The listing builds one solid part. Answer for the finished solid, in the listing's coordinates (mm). Round coordinates to 2 decimals unless told otherwise and drop trailing zeros. Order: outer loops, then holes, each group sorted by start corner. A loop starts at its lowest first (then second) coordinate and runs counter-clockwise, first axis right, second up. Notation, with made-up numbers: (-37.5, -34.75) -> (16.5, -34.75) arc R19 cw to (16.5, -7.75) -> close; hole circle Ø9 at (63.5, -33). An arc over 180 degrees is marked (long way). Answer in a Markdown table with one row per item. Add a question column.
```python
from build123d import *

# Parameters (mm, degrees)
F0_R     = 1.5875
F0_W     = 152.4
F0_H     = 3.175
F1_DEPTH = 3.175
F2_DEPTH = 6.35
F3_DEPTH = 12.7


# Not quite as in the source:
# - a feature names something its author has since deleted; it is built from what else it names


with BuildPart() as f1:
    # F0 (on Top) → F1 (new body)
    with BuildSketch(Plane.XY):
        with BuildLine():
            Line((76.2, -63.5), (76.2, 60.325))
            Line((76.2, 60.325), (-76.2, 60.325))
            Line((-76.2, 60.325), (-76.2, -63.5))
            Line((-76.2, -63.5), (-76.2, -73.025))
            Line((-76.2, -73.025), (-12.7, -73.025))
            ThreePointArc((-12.7, -73.025), (0, -85.725), (12.7, -73.025))
            Line((12.7, -73.025), (76.2, -73.025))
            Line((76.2, -73.025), (76.2, -63.5))
        make_face()
        with Locations((0, -73.025)):
            Circle(F0_R, mode=Mode.SUBTRACT)
        Polygon((3.175, -50.8), (0, -63.5), (-3.175, -50.8), align=None, mode=Mode.SUBTRACT)
        with BuildLine():
            ThreePointArc((-49.8535963292, 27.0824817792), (-54.4870485305, 34.7644782938), (-46.0375, 31.75))
            ThreePointArc((-46.0375, 31.75), (-46.7742676703, 29.2054203766), (-48.7566120041, 27.4481432208))
            ThreePointArc((-48.7566120041, 27.4481432208), (-45.0579989552, 28.2917059724), (-41.275, 28.575))
            Line((-41.275, 28.575), (41.275, 28.575))
            ThreePointArc((41.275, 28.575), (45.0579989552, 28.2917059724), (48.7566120041, 27.4481432208))
            ThreePointArc((48.7566120041, 27.4481432208), (48.2554203766, 35.7757323297), (55.5625, 31.75))
            ThreePointArc((55.5625, 31.75), (53.8144782938, 28.0629514695), (49.8535963292, 27.0824817792))
            ThreePointArc((49.8535963292, 27.0824817792), (62.0482562055, 17.7911495141), (66.675, 3.175))
            Line((66.675, 3.175), (66.675, -15.875))
            ThreePointArc((66.675, -15.875), (63.3002757063, -28.525977435), (54.0728559007, -37.8152571622))
            ThreePointArc((54.0728559007, -37.8152571622), (55.1742646512, -39.3915948361), (55.5625, -41.275))
            ThreePointArc((55.5625, -41.275), (50.5724196506, -46.0320593264), (46.0592502637, -40.8203592761))
            ThreePointArc((46.0592502637, -40.8203592761), (43.6779018277, -41.1610843708), (41.275, -41.275))
            Line((41.275, -41.275), (-41.275, -41.275))
            ThreePointArc((-41.275, -41.275), (-43.6779018277, -41.1610843708), (-46.0592502637, -40.8203592761))
            ThreePointArc((-46.0592502637, -40.8203592761), (-46.0429406736, -41.0474196506), (-46.0375, -41.275))
            ThreePointArc((-46.0375, -41.275), (-52.6834051639, -45.6492646512), (-54.0728559007, -37.8152571622))
            ThreePointArc((-54.0728559007, -37.8152571622), (-63.3002757063, -28.525977435), (-66.675, -15.875))
            Line((-66.675, -15.875), (-66.675, 3.175))
            ThreePointArc((-66.675, 3.175), (-62.0482562055, 17.7911495141), (-49.8535963292, 27.0824817792))
        make_face(mode=Mode.SUBTRACT)
        Polygon((-3.175, 38.1), (0, 50.8), (3.175, 38.1), align=None, mode=Mode.SUBTRACT)
        with Locations((0, 61.9125)):
            Rectangle(F0_W, F0_H)
        with BuildLine():
            ThreePointArc((-48.7566120041, 27.4481432208), (-46.7742676703, 29.2054203766), (-46.0375, 31.75))
            ThreePointArc((-46.0375, 31.75), (-54.4870485305, 34.7644782938), (-49.8535963292, 27.0824817792))
            ThreePointArc((-49.8535963292, 27.0824817792), (-49.3071852568, 27.2715557705), (-48.7566120041, 27.4481432208))
        make_face()
        with Locations((-50.8, 31.75)):
            Circle(F0_R, mode=Mode.SUBTRACT)
        with BuildLine():
            ThreePointArc((55.5625, 31.75), (48.2554203766, 35.7757323297), (48.7566120041, 27.4481432208))
            ThreePointArc((48.7566120041, 27.4481432208), (49.3071852568, 27.2715557705), (49.8535963292, 27.0824817792))
            ThreePointArc((49.8535963292, 27.0824817792), (53.8144782938, 28.0629514695), (55.5625, 31.75))
        make_face()
        with Locations((50.8, 31.75)):
            Circle(F0_R, mode=Mode.SUBTRACT)
        with BuildLine():
            ThreePointArc((54.0728559007, -37.8152571622), (50.1935354163, -39.6577611103), (46.0592502637, -40.8203592761))
            ThreePointArc((46.0592502637, -40.8203592761), (50.5724196506, -46.0320593264), (55.5625, -41.275))
            ThreePointArc((55.5625, -41.275), (55.1742646512, -39.3915948361), (54.0728559007, -37.8152571622))
        make_face()
        with Locations((50.8, -41.275)):
            Circle(F0_R, mode=Mode.SUBTRACT)
        with BuildLine():
            ThreePointArc((-46.0592502637, -40.8203592761), (-50.1935354163, -39.6577611103), (-54.0728559007, -37.8152571622))
            ThreePointArc((-54.0728559007, -37.8152571622), (-52.6834051639, -45.6492646512), (-46.0375, -41.275))
            ThreePointArc((-46.0375, -41.275), (-46.0429406736, -41.0474196506), (-46.0592502637, -40.8203592761))
        make_face()
        with Locations((-50.8, -41.275)):
            Circle(F0_R, mode=Mode.SUBTRACT)
    extrude(amount=F1_DEPTH)

    # F0 (on Top) → F2 (join)
    with BuildSketch(Plane.XY):
        with BuildLine():
            ThreePointArc((-46.0592502637, -40.8203592761), (-50.1935354163, -39.6577611103), (-54.0728559007, -37.8152571622))
            ThreePointArc((-54.0728559007, -37.8152571622), (-52.6834051639, -45.6492646512), (-46.0375, -41.275))
            ThreePointArc((-46.0375, -41.275), (-46.0429406736, -41.0474196506), (-46.0592502637, -40.8203592761))
        make_face()
        with Locations((-50.8, -41.275)):
            Circle(F0_R, mode=Mode.SUBTRACT)
        with BuildLine():
            ThreePointArc((-48.7566120041, 27.4481432208), (-46.7742676703, 29.2054203766), (-46.0375, 31.75))
            ThreePointArc((-46.0375, 31.75), (-54.4870485305, 34.7644782938), (-49.8535963292, 27.0824817792))
            ThreePointArc((-49.8535963292, 27.0824817792), (-49.3071852568, 27.2715557705), (-48.7566120041, 27.4481432208))
        make_face()
        with Locations((-50.8, 31.75)):
            Circle(F0_R, mode=Mode.SUBTRACT)
        with BuildLine():
            ThreePointArc((54.0728559007, -37.8152571622), (50.1935354163, -39.6577611103), (46.0592502637, -40.8203592761))
            ThreePointArc((46.0592502637, -40.8203592761), (50.5724196506, -46.0320593264), (55.5625, -41.275))
            ThreePointArc((55.5625, -41.275), (55.1742646512, -39.3915948361), (54.0728559007, -37.8152571622))
        make_face()
        with Locations((50.8, -41.275)):
            Circle(F0_R, mode=Mode.SUBTRACT)
        with BuildLine():
            ThreePointArc((55.5625, 31.75), (48.2554203766, 35.7757323297), (48.7566120041, 27.4481432208))
            ThreePointArc((48.7566120041, 27.4481432208), (49.3071852568, 27.2715557705), (49.8535963292, 27.0824817792))
            ThreePointArc((49.8535963292, 27.0824817792), (53.8144782938, 28.0629514695), (55.5625, 31.75))
        make_face()
        with Locations((50.8, 31.75)):
            Circle(F0_R, mode=Mode.SUBTRACT)
    extrude(amount=F2_DEPTH)

    # F0 (on Top) → F3 (join)
    with BuildSketch(Plane.XY):
        with Locations((0, 61.9125)):
            Rectangle(F0_W, F0_H)
    extrude(amount=F3_DEPTH)


solid = f1.part
```
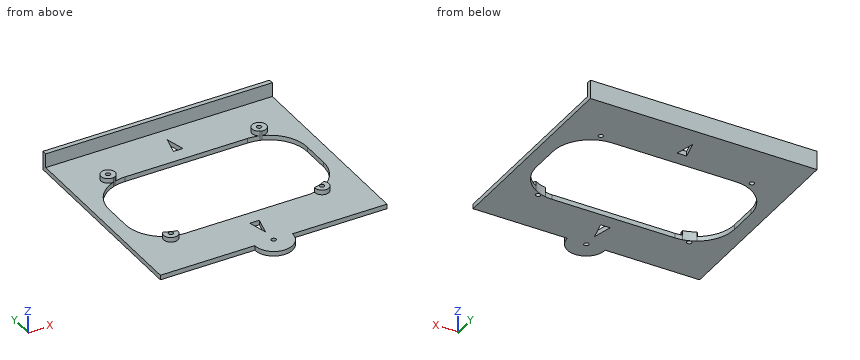
1. The part is cut by section B-B (x = -15). Give the vertices of the cut face in (y, z) (3 decimals), then the cut area to 3 significant figures.
2. The part is cut by section A-A (y = -11.5). Give the vertices of the cut face in (x, z) (3 decimals), then the cut area to 3 significant figures.
3. Straight lines are drawn through the part: line 1 along Y through (x, z) = (-50, 3.5) (3 decimals); line 2 along Y through (x, z) = (-50.5, 5.25) (3 decimals); line 3 along Y through (x, z) = (-14.5, 1) (3 decimals). For each, find the intervals that lie inside material, in ascending order.
4. The part is cut by section C-C (y = 22.5). Give the vertices of the cut face in (x, z) (3 decimals), then the cut area to 3 significant figures.
5. Each of these flat-tipped pins is pushed along its axis until it touches: pin 1 (10.5 mm diameter, centred on x = -51.5, y = 32.5, fed in from +Z); pin 2 (3.5 mm diameter, centred on x = -8.5, z = 2, fed in from -Y); pin 3 (1.6 mm diameter, centred on x = 45, z = 2, fed in from -Y) (3 decimals). Where does it stop, or does it pass through?
Report:
| question | item | result |
|---|---|---|
| 1 | outline | (-73.025, 0) -> (-41.275, 0) -> (-41.275, 3.175) -> (-73.025, 3.175) -> close; (28.575, 0) -> (63.5, 0) -> (63.5, 12.7) -> (60.325, 12.7) -> (60.325, 3.175) -> (28.575, 3.175) -> close |
| 1 | area | 242 mm^2 |
| 2 | outline | (-76.2, 0) -> (-66.675, 0) -> (-66.675, 3.175) -> (-76.2, 3.175) -> close; (66.675, 0) -> (76.2, 0) -> (76.2, 3.175) -> (66.675, 3.175) -> close |
| 2 | area | 60.5 mm^2 |
| 3 | line 1 | y = -45.97 to -42.646, -39.904 to -39.729, 27.055 to 30.379, 33.121 to 36.445, 60.325 to 63.5 |
| 3 | line 2 | y = -46.028 to -42.834, -39.716 to -39.541, 26.997 to 30.191, 33.309 to 36.503, 60.325 to 63.5 |
| 3 | line 3 | y = -73.025 to -41.275, 28.575 to 63.5 |
| 4 | outline | (-76.2, 0) -> (-57.758, 0) -> (-57.758, 3.175) -> (-76.2, 3.175) -> close; (57.758, 0) -> (76.2, 0) -> (76.2, 3.175) -> (57.758, 3.175) -> close |
| 4 | area | 117 mm^2 |
| 5 | pin 1 | stops at z = 6.35 |
| 5 | pin 2 | stops at y = -83.78 |
| 5 | pin 3 | stops at y = -73.025 |
